Read the model definition and answer for the solid it produces. Units are mm, in the model's axes. Coordinates: 2 decimals unless noted, no trailing zeros.
from build123d import *

# Parameters (mm, degrees)
F0_R     = 3.302
F0_R_2   = 2.286
F0_R_3   = 9.017
F0_R_4   = 14.2875
F1_DEPTH = 5.08


with BuildPart() as f1:
    # F0 (on Front) → F1 (new body)
    with BuildSketch(Plane.XZ):
        Polygon((530.29324, 50.937387), (-206.30676, 50.937387), (-206.30676, 0.137387), (-206.30676, -50.662613), (530.29324, -50.662613), align=None)
        with Locations((-193.60676, -37.962613)):
            Circle(F0_R, mode=Mode.SUBTRACT)
        with Locations((-31.68176, -43.042613)):
            Circle(F0_R_2, mode=Mode.SUBTRACT)
        with Locations((-140.26676, -34.152613)):
            Circle(F0_R, mode=Mode.SUBTRACT)
        with Locations((-114.86676, -34.152613)):
            Circle(F0_R, mode=Mode.SUBTRACT)
        with Locations((34.99324, -37.962613)):
            Circle(F0_R, mode=Mode.SUBTRACT)
        with Locations((60.39324, -37.962613)):
            Circle(F0_R, mode=Mode.SUBTRACT)
        with Locations((-193.60676, -12.562613)):
            Circle(F0_R, mode=Mode.SUBTRACT)
        with Locations((-59.62176, -16.372613)):
            Circle(F0_R_2, mode=Mode.SUBTRACT)
        with Locations((-31.68176, -16.372613)):
            Circle(F0_R_3, mode=Mode.SUBTRACT)
        with Locations((-6.28176, -16.372613)):
            Circle(F0_R_2, mode=Mode.SUBTRACT)
        with Locations((301.69324, -43.042613)):
            Circle(F0_R_2, mode=Mode.SUBTRACT)
        with Locations((286.45324, -37.962613)):
            Circle(F0_R, mode=Mode.SUBTRACT)
        with Locations((311.85324, -37.962613)):
            Circle(F0_R, mode=Mode.SUBTRACT)
        with Locations((517.59324, -41.090906)):
            Circle(F0_R, mode=Mode.SUBTRACT)
        with Locations((273.75324, -16.372613)):
            Circle(F0_R_2, mode=Mode.SUBTRACT)
        with Locations((301.69324, -16.372613)):
            Circle(F0_R_3, mode=Mode.SUBTRACT)
        with Locations((327.09324, -16.372613)):
            Circle(F0_R_2, mode=Mode.SUBTRACT)
        with Locations((517.59324, -15.690906)):
            Circle(F0_R, mode=Mode.SUBTRACT)
        with Locations((-193.60676, 12.837387)):
            Circle(F0_R, mode=Mode.SUBTRACT)
        with Locations((-31.68176, 10.297387)):
            Circle(F0_R_2, mode=Mode.SUBTRACT)
        with Locations((-155.50676, 25.537387)):
            Circle(F0_R_4, mode=Mode.SUBTRACT)
        with Locations((136.59324, 25.537387)):
            Circle(F0_R_4, mode=Mode.SUBTRACT)
        with Locations((-193.60676, 38.237387)):
            Circle(F0_R, mode=Mode.SUBTRACT)
        with Locations((34.99324, 38.237387)):
            Circle(F0_R, mode=Mode.SUBTRACT)
        with Locations((60.39324, 38.237387)):
            Circle(F0_R, mode=Mode.SUBTRACT)
        with Locations((301.69324, 10.297387)):
            Circle(F0_R_2, mode=Mode.SUBTRACT)
        with Locations((517.59324, 9.709094)):
            Circle(F0_R, mode=Mode.SUBTRACT)
        with Locations((428.69324, 25.537387)):
            Circle(F0_R_4, mode=Mode.SUBTRACT)
        with Locations((286.45324, 38.237387)):
            Circle(F0_R, mode=Mode.SUBTRACT)
        with Locations((311.85324, 38.237387)):
            Circle(F0_R, mode=Mode.SUBTRACT)
        with Locations((517.59324, 38.237387)):
            Circle(F0_R, mode=Mode.SUBTRACT)
    extrude(amount=F1_DEPTH)


solid = f1.part
Q1. Flat-ended cylindrical pins translate along their axes: pin 1 Ø20.5 at (x, z) = (-31.68, -16.37) entering from -Y; pin 2 Ø4 at (x, z) = (517.59, -41.09) entering from +Y. Find the tip coordinate at first contact, or state that the pin passes through.
Findings below:
pin 1: stops at y = -5.08
pin 2: passes through
Q2. A cutting plane is placed at A-A (y = -1.1). Count the separate pieces of the cut face and the enclosed holes in it, then the cut area to 3 significant figures.
Findings below:
separate pieces: 1
enclosed holes: 31
area: 71,700 mm2
Q3. Straight lines are drawn through the part: probe 1 along X at (y, z) = (-1.7, 29); probe 2 along X at (y, z) = (-3.7, 19); probe 3 along X at (y, z) = (-1.7, -44.5). For each, find the intervals that lie inside material, in ascending order.
Findings below:
probe 1: x = -206.31 to -169.37, -141.65 to 122.73, 150.45 to 414.83, 442.55 to 530.29
probe 2: x = -206.31 to -168.21, -142.8 to 123.89, 149.3 to 415.99, 441.4 to 530.29
probe 3: x = -206.31 to -33.44, -29.92 to 299.93, 303.45 to 530.29
Q4. Determine the mould class of faces 1 (the face through (157, -5.08, 1)), 2 (the face through (-40.69, -2.5, -15.98)) for opening direction Z: +Z half, -Z half, draft (parallel to the pull), parting line (faces both ways), or undercut.
Findings below:
face 1: draft
face 2: undercut
